For this review, take the finished solid that the model builds, in its own axes (mm). Face numbers are marked on the shaded views. A direction names the side the tool comes from. Coordinates: 2 decimals unless noted, no trailing zeros. Loops run counter-clockwise (first coordinate to the right, second up) from the corner with the lowest first, then second, coordinate; pieces in that order, holes last. Notation, with made-up numbers: M 41,21 L 81,21 A20 cw 81,45 Z; hole C 42,29 d6. An arc over 180 degrees is marked long. Use one line per item in the form item = value.
```python
from build123d import *

# Parameters (mm, degrees)
SKETCH1_W           = 10
SKETCH1_H           = 300
BOSS_EXTRUDE3_START = 8
SKETCH4_R           = 18
SKETCH4_R_2         = 10
BOSS_EXTRUDE3_DEPTH = 8
CHAMFER1_SIZE       = 1


with BuildPart() as part:
    # Sketch1 → Revolve1 (revolve)
    with BuildSketch(Plane.XY):
        with Locations((-7.916666667, -11.875)):
            Rectangle(SKETCH1_W, SKETCH1_H)
    revolve(axis=Axis((-2.916666667, 138.125, 0), (0, -1, 0)))

    # Sketch4 → Boss-Extrude3 (add)
    with BuildSketch(Plane(origin=(0, 80, 0), x_dir=(1, 0, 0), z_dir=(0, 1, 0)).offset(BOSS_EXTRUDE3_START)):
        with Locations(Location((-2.916666667, 0, 0), (0, 0, 270))):
            Circle(SKETCH4_R)
        with Locations(Location((-2.916666667, 0, 0), (0, 0, 180))):
            Circle(SKETCH4_R_2, mode=Mode.SUBTRACT)
    extrude(amount=-BOSS_EXTRUDE3_DEPTH)

    # Chamfer1
    chamfer1_edges = [part.edges().sort_by_distance(p)[0] for p in [
        (-2.916666667, 88, -18),
        (-2.916666667, 80, -18),
    ]]
    chamfer(chamfer1_edges, length=CHAMFER1_SIZE)


solid = part.part
```
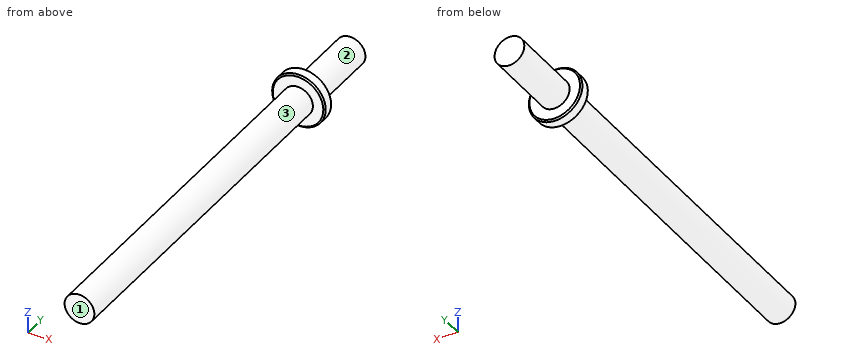
1. Consider section A-A on z = 0. Write out the cut boundary in (x, y) (3 decimals), plus the area to 3 significant figures.
Computed values:
outline = M -20.917,81 L -19.917,80 L -12.917,80 L -12.917,-161.875 L 7.083,-161.875 L 7.083,80 L 14.083,80 L 15.083,81 L 15.083,87 L 14.083,88 L 7.083,88 L 7.083,138.125 L -12.917,138.125 L -12.917,88 L -19.917,88 L -20.917,87 Z
area = 6,130 mm2
2. Tool access review of the marked faces 1, 2 and 3: name each direction out of +Z, -Z, +X, -X, +Y, -Y from which nothing blocks a thin tool from reaching the whole face with its end or side.
Computed values:
face_1 = +Z, -Z, +X, -X, -Y
face_2 = +Y
face_3 = -Y
3. Wall thickness on line 1 along Y through (x, z) = (-5.5, 10); line 2 along X through (y, z) = (-13.5, -1); line 3 along Z through (x, y) = (-4, 5): over which ranges is each line inside the solid? List them lowest first. Write a range as from..to.
Computed values:
line_1 = 80..88
line_2 = -12.87..7.03
line_3 = -9.94..9.94
4. Consider section B-B on y = 106. Write out the cut boundary in (x, z).
Computed values:
outline = C -2.92,0 d20
5. For pin 1 Ø10 at (x, y) = (6, -70.5) entering from +Z; pin 2 Ø3 at (x, z) = (-6, 13) entering from +Y; pin 3 Ø8 at (x, z) = (2.5, -10.5) entering from +Y (3 decimals); pin 4 Ø1 at (y, z) = (-54.5, 9.5) entering from +X, all flat-tipped, find the tip position at first contact; note any pin that passes through.
Computed values:
pin_1 = 9.2
pin_2 = 88
pin_3 = 138.125
pin_4 = 1.44
